from build123d import *

# Parameters (mm, degrees)
SKETCH_1_R      = 10
SKETCH_1_R_2    = 8
EXTRUDE_1_DEPTH = 24.2
SKETCH_2_R      = 10
EXTRUDE_2_DEPTH = 2
SKETCH_3_R      = 3
EXTRUDE_3_DEPTH = 24.2


with BuildPart() as part:
    # 草图1 → 凸台-拉伸1 (new body)
    with BuildSketch(Plane.XY):
        Circle(SKETCH_1_R)
        Circle(SKETCH_1_R_2, mode=Mode.SUBTRACT)
    extrude(amount=EXTRUDE_1_DEPTH)

    # 草图2 → 凸台-拉伸2 (add)
    with BuildSketch(Plane.XY.offset(24.2)):
        Circle(SKETCH_2_R)
    extrude(amount=EXTRUDE_2_DEPTH)

    # 草图3 → 凸台-拉伸3 (add)
    with BuildSketch(Plane(origin=(0, 0, 24.2), x_dir=(-1, 0, 0), z_dir=(0, 0, -1))):
        with Locations(Location((0, 0, 0), (0, 0, 180))):
            Circle(SKETCH_3_R)
    extrude(amount=EXTRUDE_3_DEPTH)


solid = part.part
Could you check a few things on this model? Use its own coordinates, in mm. A direction names the side the tool comes from. Coordinates: 2 decimals unless noted, no trailing zeros. Order: outer loops, then holes, each group sorted by start corner. A loop starts at its lowest first (then second) coordinate and runs counter-clockwise, first axis right, second up.
Q1. Which directions (+Z, -Z, +X, -X, +Y, -Y) give clear straight access to the entire face, cutting with the end or side of a thin tool? Please do faces 4 (the cylindrical face through (-1.73, -7.81, 11.93)), 5 (the flat face through (0, 8.2, 0)).
Q2. Suppose I cut it at D-D on y = 5. Please give me the cut outline in (x, z) (3 decimals), and give its area (3 significant figures).
Q3. Suppose I cut it at B-B on x = 0. Please give me the cut outline in (y, z), and give its area (3 significant figures).
Q4. Will these pins go through, and if not, where does the flat tip stop? pin 1 (6 mm diameter, centred on y = -8, z = 17.5, fed in from +X); pin 2 (3 mm diameter, centred on y = 7, z = 15, fed in from -X); pin 3 (1 mm diameter, centred on y = -4.5, z = 17.5, fed in from -X).
Q5. Please list where these lines run through material, in increasing order: L1, parallel to Y at x = 0, z = 19.5; L2, parallel to X at y = -0.25, z = 16.75; L3, parallel to Z at x = -5.75, y = -2.
Q6. Thinking about a two-plate mould opening in Y: for faces 1 (the flat face through (0, 0, 0)), 2 (the cylindrical face through (-2.17, -9.76, 12.92)), 3 (the flat face through (3.4, 0.1, 24.2)), which applies, released by +Y, released by -Y, zero draft, split by the parting line, or undercut?
Q7. Suppose I cut it at A-A on z = 2.25. Please give me the cut outline in (x, y), and give its area (3 significant figures).
Answer:
1. face 4: -Z
1. face 5: -Z, +X, -X, +Y, -Y
2. outline: (-8.66, 0) - (-6.245, 0) - (-6.245, 24.2) - (6.245, 24.2) - (6.245, 0) - (8.66, 0) - (8.66, 26.2) - (-8.66, 26.2) - close
2. area: 152 mm2
3. outline: (-10, 0) - (-8, 0) - (-8, 24.2) - (-3, 24.2) - (-3, 0) - (3, 0) - (3, 24.2) - (8, 24.2) - (8, 0) - (10, 0) - (10, 26.2) - (-10, 26.2) - close
3. area: 282 mm2
4. pin 1: stops at x = 8.66
4. pin 2: stops at x = -8.35
4. pin 3: stops at x = -9.17
5. L1: y = -10 to -8, -3 to 3, 8 to 10
5. L2: x = -10 to -8, -2.99 to 2.99, 8 to 10
5. L3: z = 24.2 to 26.2
6. face 1: zero draft
6. face 2: split by the parting line
6. face 3: undercut
7. outline: circle Ø20 at (0, 0); circle Ø6 at (0, 0); hole circle Ø16 at (0, 0)
7. area: 141 mm2
